Part print with two shaded views. Sizes in mm from the minimum x, y, z corner. A direction names the side the tool comes from. Round coordinates to 2 decimals unless told otherwise and drop trailing zeros. Write each loop counter-clockwise with the first axis right and the second up, starting at its lowest first coordinate (ties: lowest second). Pieces come first, ordered by that corner, then holes.
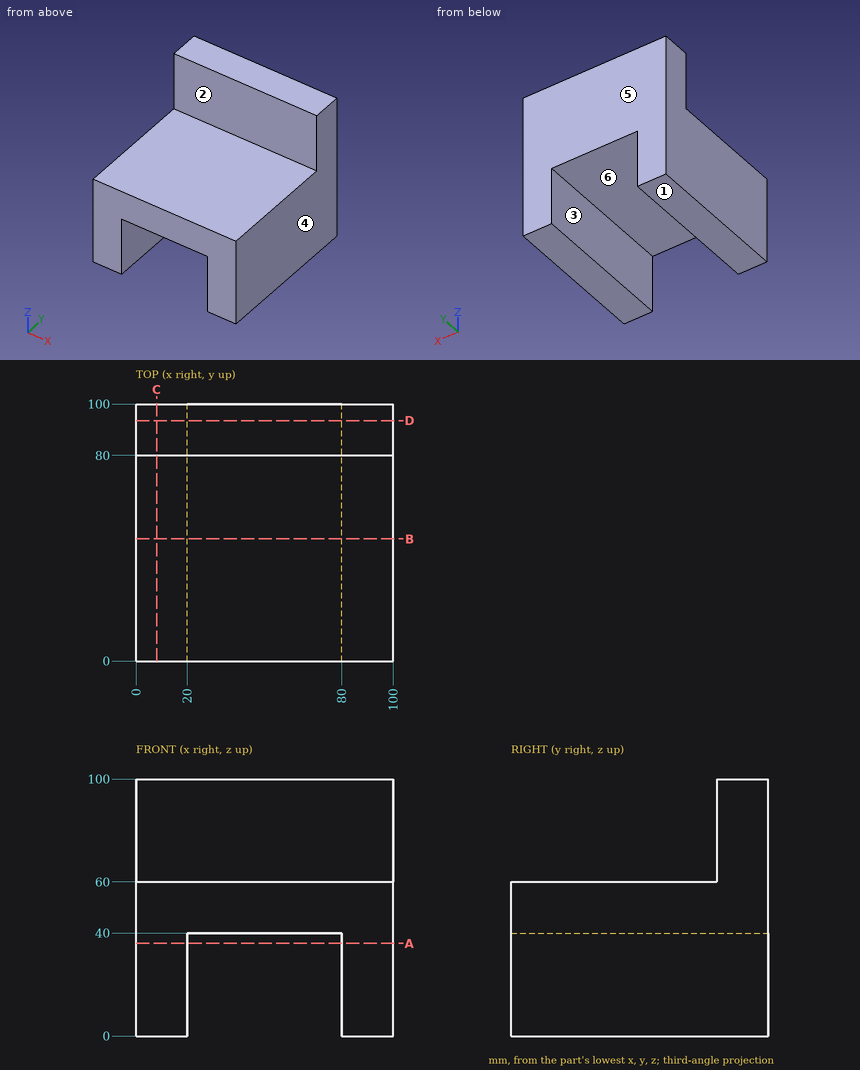
Q1. Wall check: L1, parallel to X at y = 83.5, z = 34; L2, parallel to Z at x = 40.5, y = 46; L3, parallel to Y at x = 5, z = 67. Give the ranges that are in metal, low to high.
Values follow:
L1: x = 0 to 20, 80 to 100
L2: z = 40 to 60
L3: y = 80 to 100
Q2. Which spindle directions (+Z, -Z, +X, -X, +Y, -Y) get a long thin tool onto all of the face, cutting with end or side? Do the marked faces 1, 2 and 3. Say none if no direction does.
Values follow:
face 1: -Z, +X, -X, +Y, -Y
face 2: +Z, +X, -X, -Y
face 3: -Z, +Y, -Y
Q3. Cut at D-D on y = 93.5. Write the cut outline in (x, z).
Values follow:
outline: (0, 0) - (20, 0) - (20, 40) - (80, 40) - (80, 0) - (100, 0) - (100, 100) - (0, 100) - close
Q4. Mould opens along X. For the marked faces 4, 5 and 6 say: +X half, -X half, draft (parallel to the pull), parting line (faces both ways), or undercut.
Values follow:
face 4: +X half
face 5: draft
face 6: undercut
Q5. Drop flat-ended pins along their axis: pin 1 (5 mm diameter, centred on y = 86, z = 71.5, fed in from -X); pin 2 (24 mm diameter, centred on x = 60.5, y = 41.5, fed in from +Z); pin 3 (4 mm diameter, centred on x = 33.5, y = 88.5, fed in from -Z). Give the stop position or say it passes through.
Values follow:
pin 1: stops at x = 0
pin 2: stops at z = 60
pin 3: stops at z = 40
Q6. Cut at A-A on z = 36. Write the cut outline in (x, y), plus the area to 3 significant figures.
Values follow:
outline: (0, 0) - (20, 0) - (20, 100) - (0, 100) - close; (80, 0) - (100, 0) - (100, 100) - (80, 100) - close
area: 4,000 mm2
Q7. Cut at B-B on y = 47.5. Write the cut outline in (x, z), plus the area to 3 significant figures.
Values follow:
outline: (0, 0) - (20, 0) - (20, 40) - (80, 40) - (80, 0) - (100, 0) - (100, 60) - (0, 60) - close
area: 3,600 mm2
Q8. Cut at C-C on x = 8. Write the cut outline in (y, z), plus the area to 3 significant figures.
Values follow:
outline: (0, 0) - (100, 0) - (100, 100) - (80, 100) - (80, 60) - (0, 60) - close
area: 6,800 mm2
